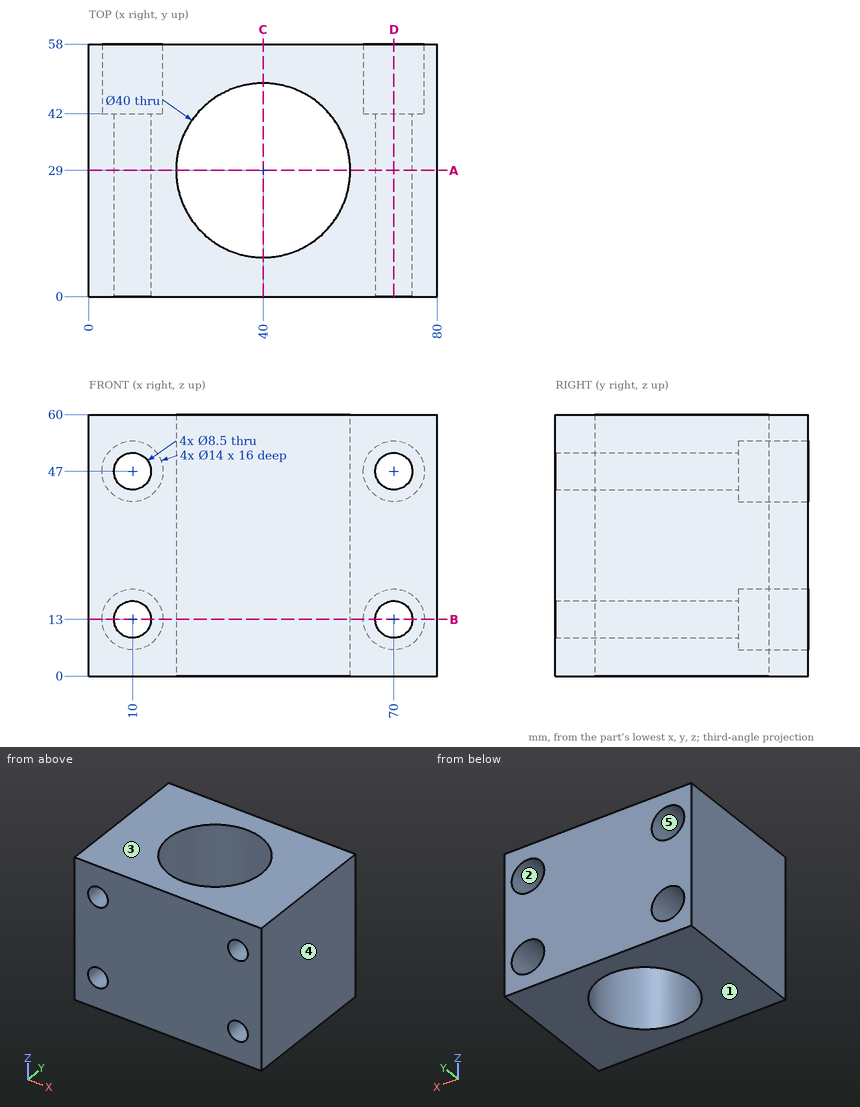
The figure shows three views and two pictorial views of one solid part (mm, origin at its lowest corner). Answer the questions. A direction names the side the tool comes from. Round coordinates to 2 decimals unless told otherwise and drop trailing zeros. Order: outer loops, then holes, each group sorted by start corner. A loop starts at its lowest first (then second) coordinate and runs counter-clockwise, first axis right, second up. Notation, with made-up numbers: M 28.25,40.25 L 37.25,40.25 A32 cw 37.25,69.25 Z; hole C 6,6 d1. An arc over 180 degrees is marked long. Put each result on its own line as item: value. Start each with the question number.
Q1. Section B-B, the plane z = 13 is taken. Write down the section's boundary in (x, y), and give its area (3 significant figures).
Q2. For a pull along Z with two mould halves and no side action, classify the marked faces 3, 4 and 5 as pulls with the +Z half, pulls with the -Z half, needs draft (parallel to the pull), parting line crosses it, or undercut.
Q3. Section C-C, the plane x = 40 is taken. Write down the section's boundary in (y, z).
Q4. Section D-D, the plane x = 70 is taken. Write down the section's boundary in (y, z), and give its area (3 significant figures).
Q5. Section A-A, the plane y = 29 is taken. Write down the section's boundary in (x, z), and give its area (3 significant figures).
Q6. A tool of negligible diameter and unlimited length cuts with its end or side. For the marked faces 1 and 2, from which of +Z, -Z, +X, -X, +Y, -Y can it reach the whole face along a straight path? Write none if from no direction.
Q7. Straight lines are drawn through the part: L1, parallel to Z at x = 70, y = 16.5; L2, parallel to Z at x = 10, y = 53.5; L3, parallel to Y at x = 40, z = 14. For each, find the intervals that lie inside material, in ascending order. Write a range as [from, to].
Q8. Flat-ended cylindrical pins translate along their axes: pin 1 (7.5 mm diameter, centred on x = 10, z = 47, fed in from -Y); pin 2 (4 mm diameter, centred on x = 72, z = 45.5, fed in from +Y). Find the tip coordinate at first contact, or state that the pin passes through.
Findings below:
1. outline: M 0,0 L 5.75,0 L 5.75,42 L 3,42 L 3,58 L 0,58 Z; M 14.25,0 L 65.75,0 L 65.75,42 L 63,42 L 63,58 L 17,58 L 17,42 L 14.25,42 Z; M 74.25,0 L 80,0 L 80,58 L 77,58 L 77,42 L 74.25,42 Z; hole C 40,29 d40
1. area: 2,220 mm^2
2. face 3: pulls with the +Z half
2. face 4: needs draft
2. face 5: undercut
3. outline: M 0,0 L 9,0 L 9,60 L 0,60 Z; M 49,0 L 58,0 L 58,60 L 49,60 Z
4. outline: M 0,0 L 58,0 L 58,6 L 42,6 L 42,8.75 L 0,8.75 Z; M 0,17.25 L 42,17.25 L 42,20 L 58,20 L 58,40 L 42,40 L 42,42.75 L 0,42.75 Z; M 0,51.25 L 42,51.25 L 42,54 L 58,54 L 58,60 L 0,60 Z
4. area: 2,320 mm^2
5. outline: M 0,0 L 20,0 L 20,60 L 0,60 Z; M 60,0 L 80,0 L 80,60 L 60,60 Z; hole C 10,13 d8.5; hole C 10,47 d8.5; hole C 70,13 d8.5; hole C 70,47 d8.5
5. area: 2,170 mm^2
6. face 1: -Z, +X, -X, +Y, -Y
6. face 2: +Y
7. L1: z = [0, 8.75], [17.25, 42.75], [51.25, 60]
7. L2: z = [0, 6], [20, 40], [54, 60]
7. L3: y = [0, 9], [49, 58]
8. pin 1: passes through
8. pin 2: stops at y = 42
